CAD build for the part. Positions are in the model's coordinates, mm. A direction names the side the tool comes from. Give positions to 0.01 mm unless a question says otherwise; leave off trailing zeros. Loops run counter-clockwise (first coordinate to the right, second up) from the corner with the lowest first, then second, coordinate; pieces in that order, holes last. Notation, with made-up numbers: M -27.75,24 L 30.25,24 A15 ccw 30.25,50 Z; hole C 29.5,-3 d2. An arc over 180 degrees is marked long. Answer as CSV lines item,"result".
from build123d import *

# Parameters (mm, degrees)
SALIENTE_EXTRUIR1_DEPTH = 3


with BuildPart() as part:
    # Croquis1 → Saliente-Extruir1 (new body)
    with BuildSketch(Plane.XY):
        with BuildLine():
            Line((14.924811557, -1.5), (10, -1.5))
            Line((10, -1.5), (10, 1.5))
            Line((10, 1.5), (14.924811557, 1.5))
            ThreePointArc((14.924811557, 1.5), (12.135254916, 8.816778784), (6.038605183, 13.730813794))
            Line((6.038605183, 13.730813794), (4.516754718, 9.047039671))
            Line((4.516754718, 9.047039671), (1.663585169, 9.974090655))
            Line((1.663585169, 9.974090655), (3.185435634, 14.657864777))
            ThreePointArc((3.185435634, 14.657864777), (-4.635254916, 14.265847744), (-11.192748309, 9.986109618))
            Line((-11.192748309, 9.986109618), (-7.208492065, 7.091378014))
            Line((-7.208492065, 7.091378014), (-8.971847822, 4.664327031))
            Line((-8.971847822, 4.664327031), (-12.956104066, 7.559058635))
            ThreePointArc((-12.956104066, 7.559058635), (-15, 0), (-12.956104066, -7.559058635))
            Line((-12.956104066, -7.559058635), (-8.971847822, -4.664327031))
            Line((-8.971847822, -4.664327031), (-7.208492065, -7.091378014))
            Line((-7.208492065, -7.091378014), (-11.192748309, -9.986109618))
            ThreePointArc((-11.192748309, -9.986109618), (-4.635254916, -14.265847744), (3.185435634, -14.657864777))
            Line((3.185435634, -14.657864777), (1.663585169, -9.974090655))
            Line((1.663585169, -9.974090655), (4.516754718, -9.047039671))
            Line((4.516754718, -9.047039671), (6.038605183, -13.730813794))
            ThreePointArc((6.038605183, -13.730813794), (12.135254916, -8.816778784), (14.924811557, -1.5))
        make_face()
    extrude(amount=SALIENTE_EXTRUIR1_DEPTH)


solid = part.part
1) Flat gauge pins, fed straight in: pin 1 (0.9 mm diameter, centred on x = 13.5, z = 1.5, fed in from -Y); pin 2 (1 mm diameter, centred on y = 10, z = 0.5, fed in from -X); pin 3 (1.5 mm diameter, centred on y = -0.5, z = 2, fed in from +X). Where does each tip first touch, or does it go through?
Answer below:
pin 1,"stops at y = -7.4"
pin 2,"stops at x = -11.19"
pin 3,"stops at x = 10"
2) Band-saw the part on A-A on x = 11. Give the cut face in (y, z), and give its area (3 significant figures).
Answer below:
outline,"M -10.2,0 L -1.5,0 L -1.5,3 L -10.2,3 Z; M 1.5,0 L 10.2,0 L 10.2,3 L 1.5,3 Z"
area,"52.2 mm^2"
3) Mould opens along X. For faces 1 (the face through (0, 0, 3)), 2 (the face through (12, -9, 1)), 3 (the face through (5.27, -11.36, 1.48)) say: +X half, -X half, draft (parallel to the pull), parting line (faces both ways), or undercut.
Answer below:
face 1,"draft"
face 2,"+X half"
face 3,"undercut"
4) Band-saw the part on C-C on y = 1. Give the cut face in (x, z), and give its area (3 significant figures).
Answer below:
outline,"M -14.97,0 L 10,0 L 10,3 L -14.97,3 Z"
area,"74.9 mm^2"
5) Band-saw the part on B-B on z = 2.4. Give the cut face in (x, y).
Answer below:
outline,"M -12.96,-7.56 L -8.97,-4.66 L -7.21,-7.09 L -11.19,-9.99 A15 ccw 3.19,-14.66 L 1.66,-9.97 L 4.52,-9.05 L 6.04,-13.73 A15 ccw 14.92,-1.5 L 10,-1.5 L 10,1.5 L 14.92,1.5 A15 ccw 6.04,13.73 L 4.52,9.05 L 1.66,9.97 L 3.19,14.66 A15 ccw -11.19,9.99 L -7.21,7.09 L -8.97,4.66 L -12.96,7.56 A15 ccw Z"
6) Band-saw the part on D-D on x = -12.5. Give the cut face in (y, z), and give its area (3 significant figures).
Answer below:
outline,"M -7.23,0 L 7.23,0 L 7.23,3 L -7.23,3 Z"
area,"43.4 mm^2"
7) Drill centre lines: line 1 (Y direction, x = -0.25, z = 1.3); line 2 (X direction, y = 11.5, z = 1.2); line 3 (X direction, y = 10.25, z = 0.9). Where is each one in solid material? Low to high. Write a range as from..to.
Answer below:
line 1,"y = -15..15"
line 2,"x = -9.63..2.16, 5.31..9.63"
line 3,"x = -10.95..1.75, 4.91..10.95"
8) Which spindle directions (+Z, -Z, +X, -X, +Y, -Y) get a long thin tool onto all of the face, cutting with end or side? Do faces 4 (the face through (-9.173, -8.518, 1.479)), 5 (the face through (-15, 0, 1)), 6 (the face through (12, 1.5, 1)). Say none if no direction does.
Answer below:
face 4,"+Z, -Z"
face 5,"+Z, -Z, -X"
face 6,"+Z, -Z, +X"
